Verification items for this drawing (mm, ordinates from the low corner). Give positions to 0.01 mm unless a question says otherwise; leave off trailing zeros. Write each loop counter-clockwise with the first axis right and the second up, starting at its lowest first coordinate (ties: lowest second). Pieces come first, ordered by that corner, then holes. Notation, with made-up numbers: (59.25, -27.75) -> (67.25, -27.75) arc R23 cw to (67.25, -5.75) -> close; hole circle Ø2 at (76, -25.5). An arc over 180 degrees is marked (long way). Answer as a JSON object with one key per item and string values.
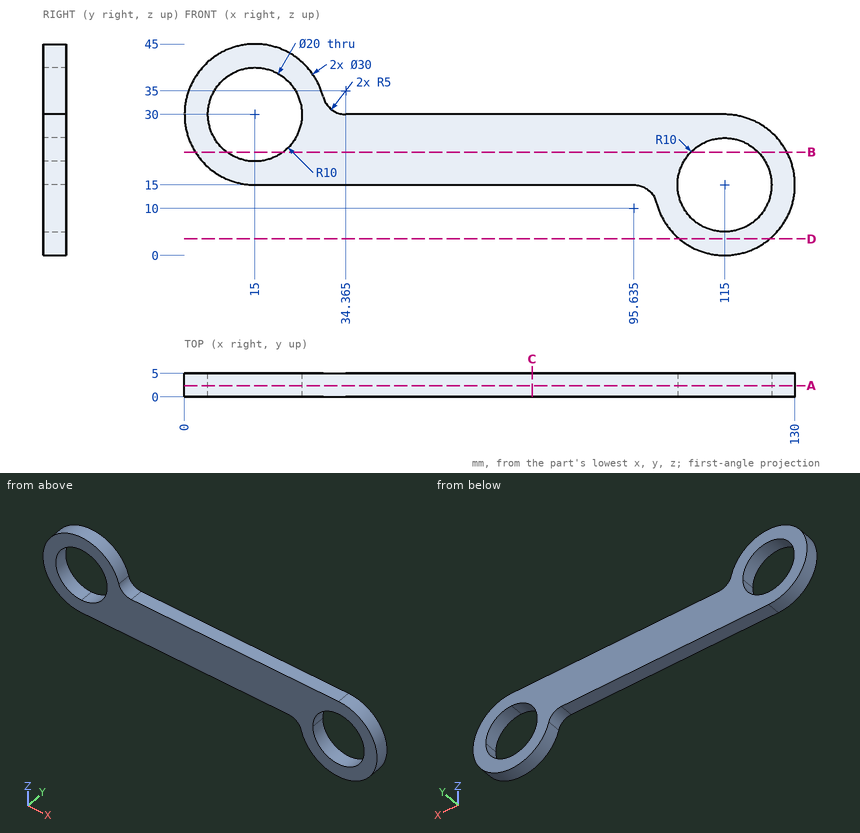
1. Sectioned sample at D-D, the plane z = 3.5. Enter the section's corners in (x, y).
Determined:
{"outline": "(105.37, 0) -> (124.63, 0) -> (124.63, 5) -> (105.37, 5) -> close"}
2. Scan lines: L1, parallel to X at y = 1.2, z = 33; L2, parallel to Z at x = 89, y = 2.7; L3, parallel to X at y = 0.7, z = 28.5 (1 decimal). Record each from-to range of solid material in increasing order. Write a range as [from, to].
Determined:
{"L1": "[0.3, 5.46], [24.54, 29.78]", "L2": "[15, 30]", "L3": "[0.1, 5.1], [24.9, 121.5]"}
3. Sectioned sample at C-C, the plane x = 74. Enter the section's corners in (y, z).
Determined:
{"outline": "(0, 15) -> (5, 15) -> (5, 30) -> (0, 30) -> close"}
4. Sectioned sample at B-B, the plane z = 22. Enter the section's corners in (x, y), plus the area to 3 significant figures.
Determined:
{"outline": "(2.31, 0) -> (9, 0) -> (9, 5) -> (2.31, 5) -> close; (21, 0) -> (107.86, 0) -> (107.86, 5) -> (21, 5) -> close; (122.14, 0) -> (128.27, 0) -> (128.27, 5) -> (122.14, 5) -> close", "area": "498 mm^2"}
5. Sectioned sample at A-A, the plane y = 2.4. Enter the section's corners in (x, z) (3 decimals).
Determined:
{"outline": "(15, 15) -> (95.635, 15) arc R5 cw to (100.476, 11.25) arc R15 ccw (long way) to (115, 30) -> (34.365, 30) arc R5 cw to (29.524, 33.75) arc R15 ccw (long way) to start; hole circle Ø20 at (15, 30); hole circle Ø20 at (115, 15)"}
6. Go/stop test with flat-tipped pins: P1, Ø2, axis at x = 33, y = 2, coming from the +Z side; P2, Ø1.5, axis at y = 3.5, z = 5, coming from the +X side; P3, Ø1.5, axis at x = 42, y = 2, coming from the -Z side. Record where each tip stops, or that it passes through.
Determined:
{"P1": "z = 30.59", "P2": "x = 126.81", "P3": "z = 15"}
